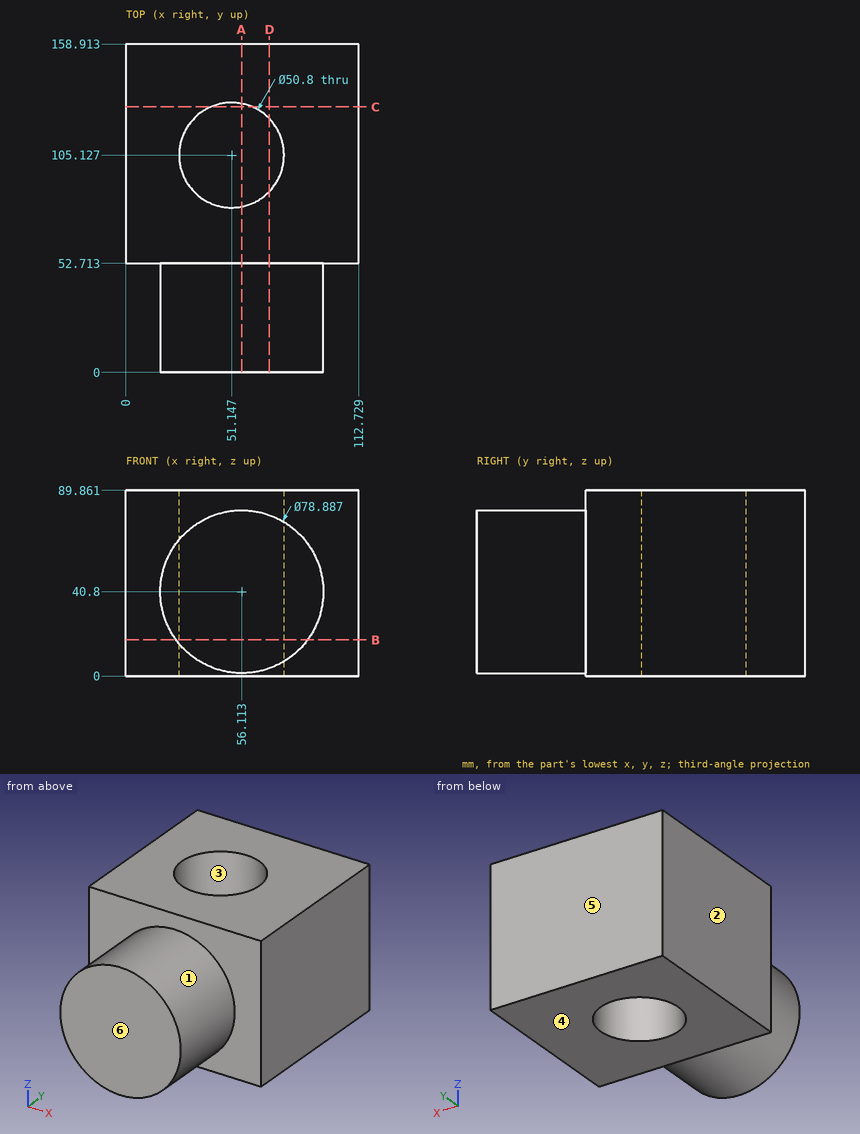
Geometry check sheet. Reference: drawing and pictorial views, mm from the part's lowest x, y, z. A direction names the side the tool comes from. Coordinates: 2 decimals unless noted, no trailing zeros. Loops run counter-clockwise (first coordinate to the right, second up) from the corner with the lowest first, then second, coordinate; pieces in that order, holes last. Notation, with made-up numbers: (36, -10.75) -> (42, -10.75) arc R18 ccw to (42, 9.25) -> close; hole circle Ø2 at (-13.75, -16.75). An arc over 180 degrees is marked (long way). Write item = value, one per line. Start each with the question number.
1. Depth check by flat-ended pin: P1, Ø1, axis at x = 31.5, y = 31, coming from the -Z side (1 decimal); P2, Ø1, axis at x = 101.5, z = 52, coming from the -Y side; P3, Ø12, axis at x = 88.5, y = 21, coming from the -Z side; P4, Ø12, axis at y = 142, z = 30.5, coming from the -X side. Enter the tip coordinate at first touch or a pass-through.
2. Draft check along Y on the marked faces 3, 4, 5 and 6. Enter one of: released by +Y, released by -Y, zero draft, split by the parting line, or undercut.
3. Tool access check on the marked faces 1 and 2. Record the directions out of +Z, -Z, +X, -X, +Y, -Y that give a thin tool (end or side, any length) a straight path to the whole face; none if there is none.
4. Section check B-B on z = 17.5. Record the cut outline in (x, y), then the cut area to 3 significant figures.
5. Section check A-A on x = 56. Record the cut outline in (y, z) (1 decimal), then the cut area to 3 significant figures.
6. Section check D-D on x = 69.5. Record the cut outline in (y, z), then the cut area to 3 significant figures.
7. Material ranges on line 1 (Y direction, x = 50, z = 80); line 2 (Y direction, x = 8, z = 68.5); line 3 (Y direction, x = 31.5, z = 34) (1 decimal), recorded low to high.
8. Section check C-C on y = 128.5. Record the cut outline in (x, z) (1 decimal).
Responses:
q1.P1 = 9.6
q1.P2 = 52.71
q1.P3 = 11.48
q1.P4 = 0
q2.face_3 = undercut
q2.face_4 = zero draft
q2.face_5 = released by +Y
q2.face_6 = released by -Y
q3.face_1 = -Y
q3.face_2 = +Z, -Z, -X, +Y, -Y
q4.outline = (0, 52.71) -> (24.29, 52.71) -> (24.29, 0) -> (87.94, 0) -> (87.94, 52.71) -> (112.73, 52.71) -> (112.73, 158.91) -> (0, 158.91) -> close; hole circle Ø50.8 at (51.15, 105.13)
q4.area = 13,300 mm2
q5.outline = (0, 1.4) -> (52.7, 1.4) -> (52.7, 0) -> (80.2, 0) -> (80.2, 89.9) -> (52.7, 89.9) -> (52.7, 80.2) -> (0, 80.2) -> close; (130.1, 0) -> (158.9, 0) -> (158.9, 89.9) -> (130.1, 89.9) -> close
q5.area = 9,220 mm2
q6.outline = (0, 3.7) -> (52.71, 3.7) -> (52.71, 0) -> (87.57, 0) -> (87.57, 89.86) -> (52.71, 89.86) -> (52.71, 77.9) -> (0, 77.9) -> close; (122.69, 0) -> (158.91, 0) -> (158.91, 89.86) -> (122.69, 89.86) -> close
q6.area = 10,300 mm2
q7.line_1 = 52.71 to 79.75, 130.5 to 158.91
q7.line_2 = 52.71 to 158.91
q7.line_3 = 0 to 89, 121.2 to 158.9
q8.outline = (0, 0) -> (41.2, 0) -> (41.2, 89.9) -> (0, 89.9) -> close; (61.1, 0) -> (112.7, 0) -> (112.7, 89.9) -> (61.1, 89.9) -> close
